Autodesk Inventor part; units mm, degrees
ref_plane "Work Plane1" through (0, 0, -2.45) normal (0, 0, 1) x (1, 0, 0)
ref_plane "YZ Plane" through (0, 0, 0) normal (1, 0, 0) x (0, 1, 0)
ref_plane "XZ Plane" through (0, 0, 0) normal (0, 1, 0) x (-1, 0, 0)
sketch "Sketch1" plane through (0, 0, 0) normal (0, 1, 0) x (-1, 0, 0)
  circle A0 centre (0, 0) radius 1.5
  circle A1 centre (0, 0) radius 2.45
  line L0 (1.118, -1) -> (-1.118, -1)
  line L1 (0.4634, -1.5) -> (-1.27, -1.5) construction
  arc A2 (-1.118, -1) -> (1.118, -1) centre (0, 0) ccw construction
  dimension "d0" = 3
  dimension "d1" = 4.9
  dimension "d2" = 0.5
extrude "Extrusion1" add sketch "Sketch1" along normal mid plane 18.5 contours L0 A0 | A1 picked at (-0.2826, -1.0791)
ref_plane "Work Plane1" through (0, 0, -2.45) normal (0, 0, 1) x (1, 0, 0)
sketch "Sketch6" plane through (0, 0, -2.45) normal (0, 0, 1) x (1, 0, 0)
  line L0 (2.5, 5.25) -> (-2.5, 5.25)
  line L1 (-2.5, 5.25) -> (-2.5, -0.75)
  line L2 (-2.5, -0.75) -> (2.5, -0.75)
  line L3 (2.5, -0.75) -> (2.5, 5.25)
  line L4 (2.45, 9.25) -> (-2.45, 9.25)
  point P0 (0, 0)
  point P1 (0, 5.25)
  dimension "d20" = 4
  dimension "d21" = 6
  dimension "d22" = 5
extrude "Extrusion6" cut sketch "Sketch6" along normal blind 0.5
properties part number "ShaftConverter"
Here's how the part is built. I have some questions about the finished solid (model axes, mm). Round coordinates to 2 decimals unless told otherwise and drop trailing zeros. Loops run counter-clockwise (first coordinate to the right, second up) from the corner with the lowest first, then second, coordinate; pieces in that order, holes last. Notation, with made-up numbers: M 84,-25.75 L 114,-25.75 A22 ccw 114,-18.75 Z; hole C 12,46 d6. An arc over 180 degrees is marked long. Write each question's results on one line, items separated by ' | '. Start each with the question number.
(1) I want a section at B-B (x = 0). Please give me the cut outline in (y, z), then the cut area to 3 significant figures.
(2) I want a section at C-C (y = -3.5). Please give me the cut outline in (x, z), then the cut area to 3 significant figures.
(3) If I drill on probe 1 along Z at (x, y) = (0, 4.25); probe 2 along Y at (x, z) = (-0.05, -2.2); probe 3 along Z at (x, y) = (0, 5.5), over which ranges is the centre line in solid material (lowest first)? Write a range as from..to.
(4) I want a section at D-D (z = 1.05). Please give me the cut outline in (x, y).
(5) I want a section at A-A (z = 0). Please give me the cut outline in (x, y), then the cut area to 4 significant figures.
(6) Will these pins go through, and if not, where does the flat tip stop? P1, Ø1.5, axis at y = 1, z = -1, coming from the +X side; P2, Ø1.5, axis at x = 2, y = -2.5, coming from the +Z side; P3, Ø2, axis at x = 2, z = -2, coming from the -Y side; P4, Ø1.5, axis at x = 1.5, y = 3.5, coming from the -Z side.
(7) Thinking about a two-plate mould opening in X: for faces 1 (the flat face through (0, 2, -1.95)), 2 (the cylindrical face through (0.5, -0.1, 2.4)), 3 (the flat face through (0, 0, -1)), which applies, pulls with the +X half, pulls with the -X half, needs draft (parallel to the pull), parting line crosses it, or undercut?
Solved:
1) outline: M -9.25,-2.45 L -0.75,-2.45 L -0.75,-1.95 L 5.25,-1.95 L 5.25,-2.45 L 9.25,-2.45 L 9.25,-1 L -9.25,-1 Z; M -9.25,1.5 L 9.25,1.5 L 9.25,2.45 L -9.25,2.45 Z | area: 41.4 mm²
2) outline: C 0,0 d4.9; hole M -1.12,-1 L 1.12,-1 A1.5 ccw long Z | area: 12.6 mm²
3) probe 1: z = -1.95..-1, 1.5..2.45 | probe 2: y = -9.25..-0.75, 5.25..9.25 | probe 3: z = -2.45..-1, 1.5..2.45
4) outline: M -2.21,-9.25 L -1.07,-9.25 L -1.07,9.25 L -2.21,9.25 Z; M 1.07,-9.25 L 2.21,-9.25 L 2.21,9.25 L 1.07,9.25 Z
5) outline: M -2.45,-9.25 L -1.5,-9.25 L -1.5,9.25 L -2.45,9.25 Z; M 1.5,-9.25 L 2.45,-9.25 L 2.45,9.25 L 1.5,9.25 Z | area: 35.15 mm²
6) P1: stops at x = 2.44 | P2: stops at z = 2.11 | P3: stops at y = -9.25 | P4: stops at z = -1.95
7) face 1: needs draft | face 2: parting line crosses it | face 3: undercut
